Read the model definition and answer for the solid it produces. Units are mm, in the model's axes. A direction names the side the tool comes from. Give positions to 0.01 mm unless a question says otherwise; leave off trailing zeros. Loops run counter-clockwise (first coordinate to the right, second up) from the corner with the lowest first, then second, coordinate; pieces in that order, holes last. Notation, with made-up numbers: (60, -6.75) - (82, -6.75) arc R20 cw to (82, 11.25) - close; hole circle Ø6 at (9.5, 18.5). An arc over 180 degrees is marked (long way). Put each result on its own line as item: value. Start each with the question number.
1. For faces 1 (the cylindrical face through (-21.202, -22.473, 0.125)), 2 (the cylindrical face through (0.213, 35.447, 0.125)), determine the directions among +Z, -Z, +X, -X, +Y, -Y from which every point of the face is accessible in a straight line to the end or side of a thin tool.
2. A cutting plane is placed at C-C, the plane x = 2. Determine the outline of the cut face in (y, z), plus the area to 3 significant figures.
3. Consider L1, parallel to X at y = -17, z = 4.25; L2, parallel to X at y = 1, z = 4; L3, parallel to Y at x = 0.5, z = -2. Determine where each line is inside the solid, lowest interval first. Write a range as from..to.
4. A cutting plane is placed at A-A, the plane z = 6.5. Determine the outline of the cut face in (x, y).
5. A cutting plane is placed at B-B, the plane y = 28.5. Determine the outline of the cut face in (x, z).
6. Given pin 1 Ø5 at (x, z) = (9, 3.5) entering from +Y; pin 2 Ø1 at (y, z) = (-27, -5.5) entering from -X; pin 3 Ø5 at (y, z) = (-20, -4) entering from +X, each flat-ended and moving along its own axis, determine where each tip first touches the part or whether it passes through.
7. For a pull along Y with two mould halves and no side action, classify faces 3 (the cylindrical face through (0.19, -29.25, 0.12)), 4 (the cylindrical face through (20.95, 21.43, 0.12)), 5 (the cylindrical face through (-33.5, -0.8, 0.1)), 6 (the cylindrical face through (24.92, -26.25, 0.12)) as released by +Y, released by -Y, zero draft, split by the parting line, or undercut.
```python
from build123d import *

# Parameters (mm, degrees)
F1_DEPTH = 8.9


with BuildPart() as f1:
    # F0 (on Top) → F1 (new body, symmetric)
    with BuildSketch(Plane.XY):
        with BuildLine():
            ThreePointArc((31.253762, 13.788255), (25.010493, 24.843211), (14.753762, 32.325853))
            ThreePointArc((14.753762, 32.325853), (0, 35.447848), (-14.753762, 32.325853))
            ThreePointArc((-14.753762, 32.325853), (-25.010493, 24.843211), (-31.253762, 13.788255))
            ThreePointArc((-31.253762, 13.788255), (-33.5, -1.029916), (-31.253762, -15.848088))
            ThreePointArc((-31.253762, -15.848088), (-25.042627, -26.128587), (-14.753762, -32.325853))
            ThreePointArc((-14.753762, -32.325853), (0, -34.552152), (14.753762, -32.325853))
            ThreePointArc((14.753762, -32.325853), (25.042627, -26.128587), (31.253762, -15.848088))
            ThreePointArc((31.253762, -15.848088), (33.5, -1.029916), (31.253762, 13.788255))
        make_face()
        with BuildLine():
            ThreePointArc((-12.606863, 27.480151), (0, 30.147848), (12.606863, 27.480151))
            ThreePointArc((12.606863, 27.480151), (21.051571, 21.319442), (26.191863, 12.217529))
            ThreePointArc((26.191863, 12.217529), (28.2, -1.029916), (26.191863, -14.277362))
            ThreePointArc((26.191863, -14.277362), (21.297489, -22.378395), (13.189863, -27.261841))
            ThreePointArc((13.189863, -27.261841), (0, -29.252152), (-13.189863, -27.261841))
            ThreePointArc((-13.189863, -27.261841), (-21.297489, -22.378395), (-26.191863, -14.277362))
            ThreePointArc((-26.191863, -14.277362), (-28.2, -1.029916), (-26.191863, 12.217529))
            ThreePointArc((-26.191863, 12.217529), (-21.051571, 21.319442), (-12.606863, 27.480151))
        make_face(mode=Mode.SUBTRACT)
    extrude(amount=F1_DEPTH, both=True)


solid = f1.part
```
Return value:
1. face 1: +Z, -Z
1. face 2: +Z, -Z, +Y
2. outline: (-34.51, -8.9) - (-29.21, -8.9) - (-29.21, 8.9) - (-34.51, 8.9) - close; (30.08, -8.9) - (35.39, -8.9) - (35.39, 8.9) - (30.08, 8.9) - close
2. area: 189 mm2
3. L1: x = -30.87..-25.12, 25.12..30.87
3. L2: x = -33.46..-28.15, 28.15..33.46
3. L3: y = -34.55..-29.25, 30.14..35.44
4. outline: (-31.25, -15.85) arc R25 ccw to (-14.75, -32.33) arc R50 ccw to (14.75, -32.33) arc R25 ccw to (31.25, -15.85) arc R50 ccw to (31.25, 13.79) arc R30 ccw to (14.75, 32.33) arc R36.42 ccw to (-14.75, 32.33) arc R30 ccw to (-31.25, 13.79) arc R50 ccw to start; hole (-26.19, -14.28) arc R19.7 ccw to (-13.19, -27.26) arc R44.7 ccw to (13.19, -27.26) arc R19.7 ccw to (26.19, -14.28) arc R44.7 ccw to (26.19, 12.22) arc R24.7 ccw to (12.61, 27.48) arc R31.12 ccw to (-12.61, 27.48) arc R24.7 ccw to (-26.19, 12.22) arc R44.7 ccw to start
5. outline: (-21.12, -8.9) - (-9.99, -8.9) - (-9.99, 8.9) - (-21.12, 8.9) - close; (9.99, -8.9) - (21.12, -8.9) - (21.12, 8.9) - (9.99, 8.9) - close
6. pin 1: stops at y = 34.86
6. pin 2: stops at x = -24.66
6. pin 3: stops at x = 30.68
7. face 3: undercut
7. face 4: undercut
7. face 5: split by the parting line
7. face 6: released by -Y
